For this review, use the dimensioned drawing (mm, ordinates from the lowest corner) and the shaded views. A direction names the side the tool comes from. Give positions to 0.01 mm unless a question says otherwise; leave off trailing zeros. Loops run counter-clockwise (first coordinate to the right, second up) from the corner with the lowest first, then second, coordinate; pieces in that order, holes last. Notation, with made-up numbers: M -11,-2 L 35,-2 A22 cw 35,11 Z; hole C -13.5,-32.5 d1. An arc over 180 degrees is marked long. Return JSON: item names as keys, results as strings.
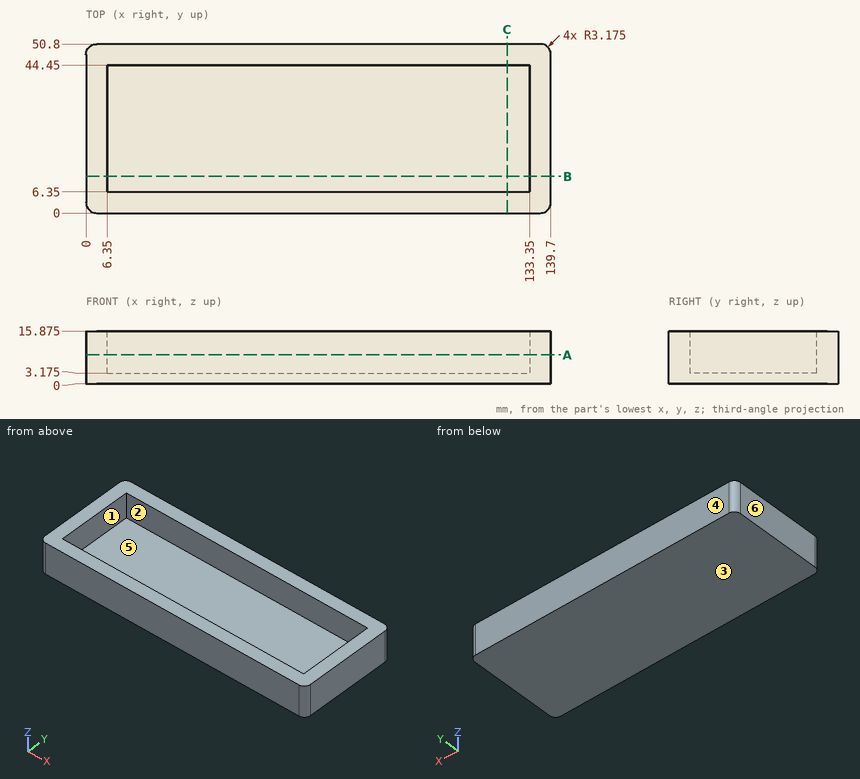
1) Wall thickness on L1, parallel to X at y = 37, z = 4.5; L2, parallel to Y at x = 50, z = 15.25: over which ranges is each line inside the solid? List them lowest first. Write a range as from..to.
From the geometry:
{"L1": "0..6.35, 133.35..139.7", "L2": "0..6.35, 44.45..50.8"}
2) Insertion check: pin 1 (10 mm diameter, centred on x = 62.5, y = 20.5, fed in from +Z) (3 decimals). The pin has a flat end and moves straight along its axis. Give the tip position at first contact, or say it passes through.
From the geometry:
{"pin 1": "z = 3.175"}
3) Consider section C-C on x = 126.5. Write out the cut boundary in (y, z) (3 decimals), then the cut area to 3 significant figures.
From the geometry:
{"outline": "M 0,0 L 50.8,0 L 50.8,15.875 L 44.45,15.875 L 44.45,3.175 L 6.35,3.175 L 6.35,15.875 L 0,15.875 Z", "area": "323 mm²"}
4) Tool access review of the marked faces 5 and 6: name each direction out of +Z, -Z, +X, -X, +Y, -Y from which nothing blocks a thin tool from reaching the whole face with its end or side.
From the geometry:
{"face 5": "+Z", "face 6": "+Z, -Z, -X, +Y, -Y"}
5) Consider section A-A on z = 8.75. Write out the cut boundary in (x, y) (3 decimals).
From the geometry:
{"outline": "M 0,3.175 A3.175 ccw 3.175,0 L 136.525,0 A3.175 ccw 139.7,3.175 L 139.7,47.625 A3.175 ccw 136.525,50.8 L 3.175,50.8 A3.175 ccw 0,47.625 Z; hole M 6.35,6.35 L 133.35,6.35 L 133.35,44.45 L 6.35,44.45 Z"}
6) Consider section B-B on y = 11. Write out the cut boundary in (x, z) (3 decimals).
From the geometry:
{"outline": "M 0,0 L 139.7,0 L 139.7,15.875 L 133.35,15.875 L 133.35,3.175 L 6.35,3.175 L 6.35,15.875 L 0,15.875 Z"}
7) The part is to be moulded in two halves that separate along Y. For the marked faces 1, 2, 3 and 4, say which applies: released by +Y, released by -Y, zero draft, split by the parting line, or undercut.
From the geometry:
{"face 1": "undercut", "face 2": "undercut", "face 3": "zero draft", "face 4": "released by +Y"}
